Input: dimensioned drawing with shaded views. Units: mm. Origin: part minimum x, y, z. Round coordinates to 2 decimals unless told otherwise and drop trailing zeros. Write each loop counter-clockwise with the first axis right and the second up, starting at its lowest first coordinate (ties: lowest second). Pieces come first, ordered by that corner, then holes. Notation, with made-up numbers: M 87.5,-36.75 L 122.5,-36.75 A19 cw 122.5,-12.75 Z; hole C 10,-31 d1. An arc over 180 degrees is marked long. Answer in a Markdown table with one row per item. Add a question column.
Item 1: Cut plane B-B on z = 44. Return loops of the section in (x, y) (1 decimal).
Item 2: Material intervals for probe 1 along X at (y, z) = (0.75, 34.5); probe 2 along X at (y, z) = (4.5, 51.5); probe 3 along Y at (x, z) = (4.75, 14), sorted ascending.
Item 3: Contact query for flat-ended pins moving along their axis: pin 1 (5 mm diameter, centred on y = 9.5, z = 21, fed in from -X); pin 2 (1.9 mm diameter, centred on x = 22.86, z = 35.03, fed in from +Y); pin 3 (3 mm diameter, centred on y = 2.5, z = 22.5, fed in from +X); pin 4 (1.5 mm diameter, centred on y = 9.5, z = 21.5, fed in from +X) (1 decimal). Output: stop coordinate, or through.
Item 4: Cut plane C-C on y = 3.5. Give the number of separate pieces and of enclosed holes in the cut face, and give its area (3 significant figures).
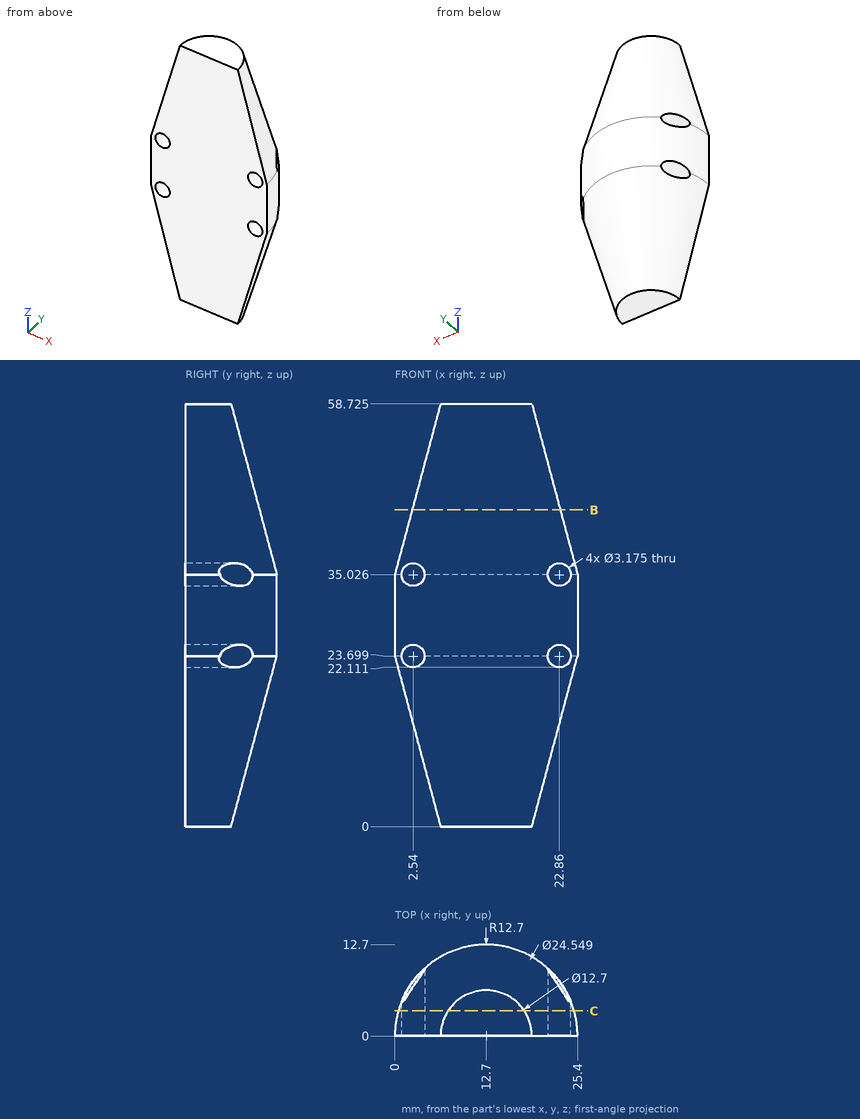
Results below:
| question | item | result |
|---|---|---|
| 1 | outline | M 2.4,0 L 23,0 A10.3 ccw Z |
| 2 | probe 1 | 0.02 to 1.04, 4.04 to 21.36, 24.36 to 25.38 |
| 2 | probe 2 | 5.74 to 19.66 |
| 2 | probe 3 | 0 to 6.23 |
| 3 | pin 1 | x = 2.8 |
| 3 | pin 2 | through |
| 3 | pin 3 | x = 25.3 |
| 3 | pin 4 | x = 21.1 |
| 4 | separate pieces | 1 |
| 4 | enclosed holes | 4 |
| 4 | area | 1,080 mm2 |
